Read the model definition and answer for the solid it produces. Units are mm, in the model's axes. A direction names the side the tool comes from. Round coordinates to 2 decimals unless told otherwise and drop trailing zeros. Loops run counter-clockwise (first coordinate to the right, second up) from the corner with the lowest first, then second, coordinate; pieces in that order, holes last. Notation, with made-up numbers: (25.25, 63.5) - (59.25, 63.5) arc R15 cw to (59.25, 68.5) - close; hole circle Ø11 at (36, -20.5). An arc over 180 degrees is marked (long way). Use CSV: the item, a comma, the result in double quotes. Start each with the question number.
1. Find section A-A (z = 0). Give the vertices of the cut face in (x, y).
2. Given pin 1 Ø1.8 at (x, z) = (0, 0) entering from -Y; pin 2 Ø1.6 at (y, z) = (5, -21.5) entering from -X; pin 3 Ø2 at (y, z) = (1.5, -17) entering from +X; pin 4 Ø1 at (y, z) = (2, -10.5) entering from -X, each flat-ended and moving along its own axis, determine where each tip first touches the part or whether it passes through.
3. Consider line 1 along Z through (x, y) = (0, 4.4); line 2 along Z through (x, y) = (0, 2.65); line 3 along Z through (x, y) = (0, 1.45). Determine where each line is inside the solid, lowest interval first.
4. Determine the mould class of faces 1 (the cylindrical face through (0.195, 2.958, -25.487)), 2 (the cylindrical face through (0, 5, -17)), 3 (the flat face through (0, 0, -10)) for opening direction X: +X half, -X half, draft (parallel to the pull), parting line (faces both ways), or undercut.
5. Find section D-D (z = -16). Give the vertices of the cut face in (x, y), and give its area (3 significant figures).
6. Find section C-C (y = 0.95). Give the vertices of the cut face in (x, z).
7. Find section B-B (x = 0). Give the vertices of the cut face in (y, z).
8. A tool of negligible diameter and unlimited length cuts with its end or side. For faces 4 (the cylindrical face through (-2.44, 2.96, 7.09)), 5 (the flat face through (-3.75, 2, -18)), 6 (the flat face through (-3, 5, -22)), 7 (the cylindrical face through (0, 5, -27)), from which of +Z, -Z, +X, -X, +Y, -Y can it reach the whole face along a straight path? Write none if from no direction.
Autodesk Inventor part; units mm, degrees
ref_plane "YZ Plane" through (0, 0, 0) normal (1, 0, 0) x (0, 1, 0)
ref_plane "XZ Plane" through (0, 0, 0) normal (0, 1, 0) x (-1, 0, 0)
ref_plane "XY Plane" through (0, 0, 0) normal (0, 0, 1) x (1, 0, 0)
sketch "Sketch1" plane through (0, 0, 0) normal (0, 1, 0) x (-1, 0, 0)
  circle A0 centre (0, 0) radius 7.5
  line L0 (0, 0) -> (0, -24) construction
  line L1 (-3.75, 0) -> (-3.75, -24)
  line L2 (3.75, -24) -> (3.75, 0)
  arc A1 (3.75, 0) -> (-3.75, 0) centre (0, 0) ccw
  arc A2 (-3.75, -24) -> (3.75, -24) centre (0, -24) ccw
  arc A3 (6.5919, -3.5773) -> (3.75, -12) centre (29.4438, -15.9785) ccw
  line L3 (0, -34.8) -> (0, 14.55)
  arc A4 (-3.75, -12) -> (-6.5919, -3.5773) centre (-29.4438, -15.9785) ccw
  circle A5 centre (0, -24) radius 1.5
  circle A6 centre (0, -20) radius 1.5
  point P0 (0, -12)
  point P1 (-6.5919, -3.5773)
  point P2 (-3.75, -12)
  dimension "d0" = 15
  dimension "d1" = 24
  dimension "d2" = 7.5
  dimension "d3" = 26
  dimension "d4" = 3
  dimension "d5" = 3
  dimension "d6" = 20
extrude "Extrusion1" add sketch "Sketch1" along normal blind 6 contours A0 L2 A1 L3 | A3 L2 A0 | L2 A2 L3 A5 A6 A0 | A0 L3 A1 L2 | L3 A1 L1 A0 | L3 A6 A5 A2 L1 A0 | A0 L1 A1 L3 | A0 L1 A4
sketch "Sketch2" plane through (0, 6, 0) normal (0, 1, 0) x (1, 0, 0)
  circle A0 centre (0, 0) radius 7.5
  arc A1 (-6.5919, 3.5773) -> (6.5919, 3.5773) centre (0, 0) ccw
  circle A2 centre (0, 20) radius 1.5
  circle A3 centre (0, 24) radius 1.5
  circle A4 centre (0, 24) radius 1.5
  line L0 (0, 20) -> (0, 24) construction
  line L1 (3, 20) -> (3, 24)
  line L2 (-3, 24) -> (-3, 20)
  arc A5 (-3, 20) -> (3, 20) centre (0, 20) ccw
  arc A6 (3, 24) -> (-3, 24) centre (0, 24) ccw
  arc A7 (-6.5919, 3.5773) -> (6.5919, 3.5773) centre (0, 0) ccw
  arc A8 (3.75, 12) -> (6.5919, 3.5773) centre (29.4438, 15.9785) ccw
  line L3 (3.75, 12) -> (3.75, 24)
  arc A9 (3.75, 24) -> (-3.75, 24) centre (0, 24) ccw
  line L4 (-3.75, 24) -> (-3.75, 12)
  arc A10 (-6.5919, 3.5773) -> (-3.75, 12) centre (-29.4438, 15.9785) ccw
  circle A11 centre (0, 20) radius 1.5
  circle A12 centre (0, 24) radius 1.5
  point P0 (0, 22)
  point P1 (-6.5919, 3.5773)
  point P2 (6.5919, 3.5773)
  dimension "d9" = 6
extrude "Extrusion2" cut sketch "Sketch2" against normal blind 2 contours A0 A10 L4 A9 L3 A8
sketch "Sketch3" plane through (0, 6, 0) normal (0, 1, 0) x (1, 0, 0)
  circle A0 centre (0, 0) radius 3
  dimension "d12" = 6
extrude "Extrusion3" cut sketch "Sketch3" against normal through all
sketch "Sketch4" plane through (0, 0, 0) normal (0, -1, 0) x (1, 0, 0)
  circle A0 centre (0, 0) radius 1.5
  circle A1 centre (0, 0) radius 3
  dimension "d15" = 3
extrude "Extrusion4" add sketch "Sketch4" against normal blind 2.5
properties part number "ServoArm" material "Stainless Steel"
Filled sheet:
1,outline,"(-7.5, 0) - (-1.5, 0) - (-1.5, 2.5) - (-3, 2.5) - (-3, 6) - (-7.5, 6) - close; (1.5, 0) - (7.5, 0) - (7.5, 6) - (3, 6) - (3, 2.5) - (1.5, 2.5) - close"
2,pin 1,"passes through"
2,pin 2,"stops at x = -3"
2,pin 3,"stops at x = 3.75"
2,pin 4,"stops at x = -4.14"
3,line 1,"z = -27 to -25.5, -22.5 to -21.5, -18.5 to -17, -7.5 to -3, 3 to 7.5"
3,line 2,"z = -27.75 to -25.5, -22.5 to -21.5, -18.5 to -3, 3 to 7.5"
3,line 3,"z = -27.75 to -25.5, -22.5 to -21.5, -18.5 to -1.5, 1.5 to 7.5"
4,face 1,"undercut"
4,face 2,"parting line"
4,face 3,"draft"
5,outline,"(-3.75, 0) - (3.75, 0) - (3.75, 4) - (-3.75, 4) - close"
5,area,"30.0 mm²"
6,outline,"(-6.59, -3.58) arc R26 cw to (-3.75, -12) - (-3.75, -24) arc R3.75 ccw to (3.75, -24) - (3.75, -12) arc R26 cw to (6.59, -3.58) arc R7.5 ccw (long way) to start; hole circle Ø3 at (0, -24); hole circle Ø3 at (0, -20); hole circle Ø3 at (0, 0)"
7,outline,"(0, -27.75) - (4, -27.75) - (4, -27) - (6, -27) - (6, -25.5) - (0, -25.5) - close; (0, -22.5) - (6, -22.5) - (6, -21.5) - (0, -21.5) - close; (0, -18.5) - (6, -18.5) - (6, -17) - (4, -17) - (4, -7.5) - (6, -7.5) - (6, -3) - (2.5, -3) - (2.5, -1.5) - (0, -1.5) - close; (0, 1.5) - (2.5, 1.5) - (2.5, 3) - (6, 3) - (6, 7.5) - (0, 7.5) - close"
8,face 4,"+Y"
8,face 5,"-Z, -X, +Y, -Y"
8,face 6,"-Z, -X, +Y"
8,face 7,"-Z, +Y"
